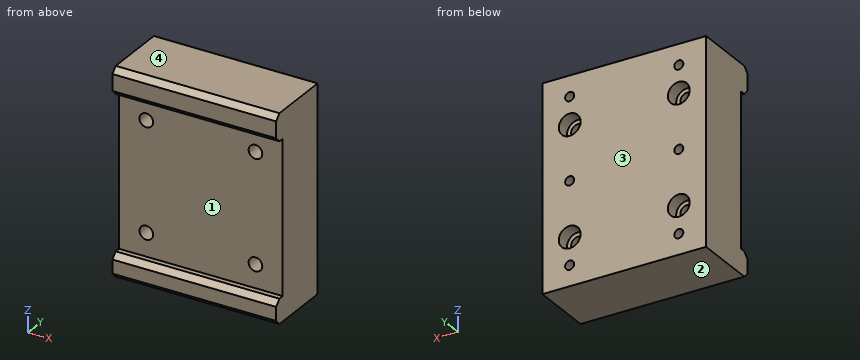
from build123d import *

# Parameters (mm, degrees)
SKETCH_1_W             = 60
SKETCH_1_H             = 75
EXTRUDE_1_DEPTH        = 25
SKETCH_2_W             = 56
SKETCH_2_H             = 4
CUT_EXTRUDE_1_DEPTH    = 100.247166206
CHAMFER_1_SIZE         = 2
SKETCH_3_R             = 4
CUT_EXTRUDE_2_DEPTH    = 5
SKETCH_4_R             = 2.5
CUT_EXTRUDE_3_DEPTH    = 99.107084352
HOLE_WIZARD_M4_1_D     = 3.3
HOLE_WIZARD_M4_1_DEPTH = 14.5
HOLE_WIZARD_M4_1_TIP   = 0.991420021


with BuildPart() as part:
    # 스케치1 → 보스-돌출1 (new body)
    with BuildSketch(Plane(origin=(0, 0, 0), x_dir=(1, 0, 0), z_dir=(0, 1, 0))):
        with Locations((30, 37.5)):
            Rectangle(SKETCH_1_W, SKETCH_1_H)
    extrude(amount=EXTRUDE_1_DEPTH)

    # 스케치2 → 컷-돌출1 (cut, through all)
    with BuildSketch(Plane(origin=(60, 0, 0), x_dir=(0, 0, -1), z_dir=(1, 0, 0))):
        with Locations((38, 2)):
            Rectangle(SKETCH_2_W, SKETCH_2_H)
    extrude(amount=-CUT_EXTRUDE_1_DEPTH, mode=Mode.SUBTRACT)

    # 모따기1
    chamfer_1_edges = [part.edges().sort_by_distance(p)[0] for p in [
        (30, 0, -10),
        (30, 0, -66),
        (30, 0, -75),
        (30, 0, 0),
    ]]
    chamfer(chamfer_1_edges, length=CHAMFER_1_SIZE)

    # 스케치3 → 컷-돌출2 (cut)
    with BuildSketch(Plane(origin=(0, 25, 0), x_dir=(1, 0, 0), z_dir=(0, 1, 0))):
        with Locations(Location((10, 57.5, 0), (0, 0, 270))):
            Circle(SKETCH_3_R)
        with Locations(Location((10, 17.5, 0), (0, 0, 270))):
            Circle(SKETCH_3_R)
        with Locations(Location((50, 57.5, 0), (0, 0, 270))):
            Circle(SKETCH_3_R)
        with Locations(Location((50, 17.5, 0), (0, 0, 270))):
            Circle(SKETCH_3_R)
    extrude(amount=-CUT_EXTRUDE_2_DEPTH, mode=Mode.SUBTRACT)

    # 스케치4 → 컷-돌출3 (cut, through all)
    with BuildSketch(Plane(origin=(0, 20, 0), x_dir=(1, 0, 0), z_dir=(0, 1, 0))):
        with Locations(Location((10, 57.5, 0), (0, 0, 270))):
            Circle(SKETCH_4_R)
        with Locations(Location((50, 57.5, 0), (0, 0, 270))):
            Circle(SKETCH_4_R)
        with Locations(Location((50, 17.5, 0), (0, 0, 270))):
            Circle(SKETCH_4_R)
        with Locations(Location((10, 17.5, 0), (0, 0, 270))):
            Circle(SKETCH_4_R)
    extrude(amount=-CUT_EXTRUDE_3_DEPTH, mode=Mode.SUBTRACT)

    # M4 나사 구멍1
    with Locations(Plane(origin=(0, 25, 0), x_dir=(1, 0, 0), z_dir=(0, 1, 0))):
        with Locations((10, 67.5), (10, 37.5), (10, 7.5), (50, 67.5), (50, 37.5), (50, 7.5)):
            Hole(HOLE_WIZARD_M4_1_D / 2, depth=HOLE_WIZARD_M4_1_DEPTH)
            with Locations((0, 0, -(HOLE_WIZARD_M4_1_DEPTH + HOLE_WIZARD_M4_1_TIP / 2))):  # 118° drill point
                Cone(0, HOLE_WIZARD_M4_1_D / 2, HOLE_WIZARD_M4_1_TIP, mode=Mode.SUBTRACT)


solid = part.part
Model file for the job. Use its own axes, mm. Face numbers are marked on the shaded views. Give positions to 0.01 mm unless a question says otherwise; leave off trailing zeros. Loops run counter-clockwise (first coordinate to the right, second up) from the corner with the lowest first, then second, coordinate; pieces in that order, holes last. Notation, with made-up numbers: (11, -38) - (25, -38) arc R26 ccw to (25, -11) - close; hole circle Ø8 at (56, 17.5). An arc over 180 degrees is marked (long way). Use one line per item in the form item = value.
(1) Drill centre lines: L1, parallel to X at y = 22.05, z = -57.5; L2, parallel to X at y = 9.75, z = -57.5; L3, parallel to Z at x = 11, y = 23.75. Where is each one in solid material? Low to high.
Determined:
L1 = 0 to 6, 14 to 46, 54 to 60
L2 = 0 to 7.5, 12.5 to 47.5, 52.5 to 60
L3 = -75 to -68.81, -66.19 to -61.37, -53.63 to -38.81, -36.19 to -21.37, -13.63 to -8.81, -6.19 to 0
(2) Cut at A-A (z = -57.5). Give the cut face in (x, y).
Determined:
outline = (0, 4) - (7.5, 4) - (7.5, 20) - (6, 20) - (6, 25) - (0, 25) - close; (12.5, 4) - (47.5, 4) - (47.5, 20) - (46, 20) - (46, 25) - (14, 25) - (14, 20) - (12.5, 20) - close; (52.5, 4) - (60, 4) - (60, 25) - (54, 25) - (54, 20) - (52.5, 20) - close
(3) Cut at D-D (x = 15.5). Give the cut face in (y, z), then the cut area to 3 significant figures.
Determined:
outline = (0, -73) - (2, -75) - (25, -75) - (25, 0) - (2, 0) - (0, -2) - (0, -8) - (2, -10) - (4, -10) - (4, -66) - (2, -66) - (0, -68) - close
area = 1,640 mm^2
(4) Cut at B-B (y = 5.25). Give the cut face in (x, z), then the cut area to 3 significant figures.
Determined:
outline = (0, -75) - (60, -75) - (60, 0) - (0, 0) - close; hole circle Ø5 at (10, -57.5); hole circle Ø5 at (10, -17.5); hole circle Ø5 at (50, -57.5); hole circle Ø5 at (50, -17.5)
area = 4,420 mm^2
(5) Cut at C-C (y = 21.25). Count the separate pieces of the cut face and the enclosed holes in it, then the cut area to 3 significant figures.
Determined:
separate_pieces = 1
enclosed_holes = 10
area = 4,250 mm^2
(6) Drop flat-ended pins along their axis: P1, Ø2.5, axis at x = 10, z = -7.5, coming from the +Y side; P2, Ø2, axis at x = 10, z = -37.5, coming from the -Y side. Give the stop position or say it passes through.
Determined:
P1 = 10.26
P2 = 4
(7) Pull direction Z, two halves, no side cores. Call the marked faces 1, 2, 3 and 4: pulls with the +Z half, pulls with the -Z half, needs draft (parallel to the pull), parting line crosses it, or undercut.
Determined:
face_1 = undercut
face_2 = pulls with the -Z half
face_3 = needs draft
face_4 = pulls with the +Z half
